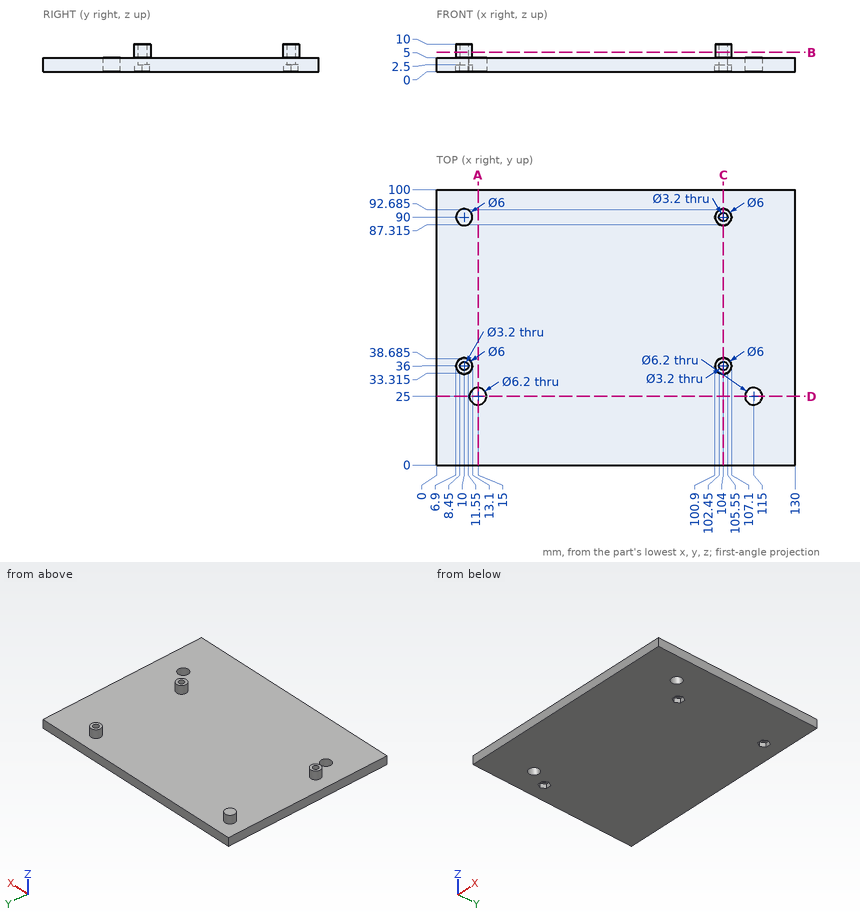
Design review of the part shown in the three views and the two pictorial views. Dimensions are in mm from the part's minimum x, y and z. Coordinates: 2 decimals unless noted, no trailing zeros. Loops run counter-clockwise (first coordinate to the right, second up) from the corner with the lowest first, then second, coordinate; pieces in that order, holes last. Notation, with made-up numbers: (-16.5, 74.25) - (29.5, 74.25) arc R28 cw to (29.5, 109.25) - close; hole circle Ø2 at (-3, -36.75). An arc over 180 degrees is marked (long way). Use a Markdown table: item, result. Add a question column.
Item 1: We need section D-D (y = 25). Give the boundary of the cut face in (x, z), and give its area (3 significant figures).
Item 2: Insertion check: pin 1 Ø1.9 at (x, y) = (10, 36) entering from +Z; pin 2 Ø0.8 at (x, z) = (103.5, 1.5) entering from -Y; pin 3 Ø3.5 at (x, y) = (104, 36) entering from -Z; pin 4 Ø12 at (x, y) = (106.5, 14.5) entering from +Z. Each pin has a flat end and moves straight along its axis. Give the tip position at first contact, or say it passes through.
Item 3: For line 1 (X direction, y = 36, z = 4.5); line 2 (Y direction, x = 15, z = 1.6); line 3 (Y direction, x = 10, z = 5.5), list the stretches that pass through material, from the lowest coordinate up.
Item 4: We need section C-C (x = 104). Give the boundary of the cut face in (y, z) (1 decimal).
Item 5: We need section B-B (z = 7). Give the boundary of the cut face in (x, y).
Item 6: We need section A-A (x = 15). Give the boundary of the cut face in (y, z), and give its area (3 significant figures).
Results list:
| question | item | result |
|---|---|---|
| 1 | outline | (0, 0) - (11.9, 0) - (11.9, 5) - (0, 5) - close; (18.1, 0) - (111.9, 0) - (111.9, 5) - (18.1, 5) - close; (118.1, 0) - (130, 0) - (130, 5) - (118.1, 5) - close |
| 1 | area | 588 mm^2 |
| 2 | pin 1 | passes through |
| 2 | pin 2 | stops at y = 0 |
| 2 | pin 3 | stops at z = 2.5 |
| 2 | pin 4 | stops at z = 5 |
| 3 | line 1 | x = 0 to 8.4, 11.6 to 102.4, 105.6 to 130 |
| 3 | line 2 | y = 0 to 21.9, 28.1 to 100 |
| 3 | line 3 | y = 33 to 34.4, 37.6 to 39, 87 to 93 |
| 4 | outline | (0, 0) - (33.3, 0) - (33.3, 2.5) - (34.4, 2.5) - (34.4, 10) - (33, 10) - (33, 5) - (0, 5) - close; (37.6, 2.5) - (38.7, 2.5) - (38.7, 0) - (87.3, 0) - (87.3, 2.5) - (88.4, 2.5) - (88.4, 10) - (87, 10) - (87, 5) - (39, 5) - (39, 10) - (37.6, 10) - close; (91.6, 2.5) - (92.7, 2.5) - (92.7, 0) - (100, 0) - (100, 5) - (93, 5) - (93, 10) - (91.6, 10) - close |
| 5 | outline | circle Ø6 at (10, 36); circle Ø6 at (10, 90); circle Ø6 at (104, 36); circle Ø6 at (104, 90); hole circle Ø3.2 at (10, 36); hole circle Ø3.2 at (104, 36); hole circle Ø3.2 at (104, 90) |
| 6 | outline | (0, 0) - (21.9, 0) - (21.9, 5) - (0, 5) - close; (28.1, 0) - (100, 0) - (100, 5) - (28.1, 5) - close |
| 6 | area | 469 mm^2 |
